Solid Edge part; units mm, degrees
sketch "Sketch1" plane through (0, 0, 0) normal (0, 0, 1) x (1, 0, 0)
  line L0 (0, 0) -> (0, 38.1)
  line L1 (0, 38.1) -> (57.15, 38.1)
  line L2 (57.15, 38.1) -> (57.15, 0)
  line L3 (57.15, 0) -> (0, 0)
  dimension "D1" = 57.15
extrude "Protrusion1" add sketch "Sketch1" along normal blind 9.525
fillet "Round_1" radius 3.175 4 edges at (0, 0, 4.7625) (0, 38.1, 4.7625) (57.15, 38.1, 4.7625) (57.15, 0, 4.7625)
hole "Hole_1" at (50.8, 12.7, 9.525) direction (0, 0, -1) diameter 4.1656 end up to next countersink diameter 9.1186 countersink angle 82
hole "Hole1" at (6.35, 12.7, 9.525) direction (0, 0, -1) diameter 4.1656 end up to next countersink diameter 9.1186 countersink angle 82
hole "Hole_3" at (47.625, 34.29, 9.525) direction (0, 0, -1) diameter 2.1565 end through all
hole "Hole2" at (9.525, 34.29, 9.525) direction (0, 0, -1) diameter 2.1565 end through all
hole "Hole_10" at (50.8, 6.35, 9.525) direction (0, 0, -1) diameter 3.3071 end up to next
hole "Hole3" at (6.35, 6.35, 9.525) direction (0, 0, -1) diameter 3.3071 end up to next
properties material "Polyethylene, low density"
CAD build for the part. Positions are in the model's coordinates, mm. Round coordinates to 2 decimals unless told otherwise and drop trailing zeros. Write each loop counter-clockwise with the first axis right and the second up, starting at its lowest first coordinate (ties: lowest second). Pieces come first, ordered by that corner, then holes. Notation, with made-up numbers: (-25, 58) - (16, 58) arc R38 ccw to (16, 96) - close; hole circle Ø4 at (15, 55.5). An arc over 180 degrees is marked (long way). Return JSON: item names as keys, results as strings. Group by question number.
Item 1: Band-saw the part on D-D on y = 6.35. List the corners of the cut face in (x, z) (3 decimals), plus the area to 3 significant figures.
Item 2: Mould opens along X. For faces 1 (the face through (57.15, 19, 5)), 2 (the face through (0, 19, 5)), 3 (the face through (4.736, 6.708, 4.829)), 4 (the face through (6.44, 14.78, 3.38)) say: +X half, -X half, draft (parallel to the pull), parting line (faces both ways), or undercut.
Item 3: Band-saw the part on A-A on y = 34.29. List the corners of the cut face in (x, z) (3 decimals).
Item 4: Probe probe 1 along X at (y, z) = (34.29, 7.5); probe 2 along X at (y, z) = (6.35, 5.5); probe 3 along Y at (x, z) = (7, 9). List the from-to ranges inside material, lowest first.
Item 5: Band-saw the part on C-C on z = 2. State how many separate pieces and enclosed holes the cut face has, plus the area to 3 significant figures.
Item 6: Flat gauge pins, fed straight in: pin 1 Ø1.3 at (x, y) = (9.525, 34.29) entering from +Z; pin 2 Ø5.5 at (x, y) = (6.35, 12.7) entering from +Z. Where does each tip first touch, or does it go through?
Item 7: Band-saw the part on B-B on x = 6.35. List the corners of the cut face in (y, z) (3 decimals).
Resolved:
{
 "1": {"outline": "(0, 0) - (4.696, 0) - (4.696, 9.525) - (0, 9.525) - close; (8.004, 0) - (49.146, 0) - (49.146, 9.525) - (8.004, 9.525) - close; (52.454, 0) - (57.15, 0) - (57.15, 9.525) - (52.454, 9.525) - close", "area": "481 mm²"},
 "2": {"face 1": "+X half", "face 2": "-X half", "face 3": "undercut", "face 4": "undercut"},
 "3": {"outline": "(0, 0) - (8.447, 0) - (8.447, 9.525) - (0, 9.525) - close; (10.603, 0) - (46.547, 0) - (46.547, 9.525) - (10.603, 9.525) - close; (48.703, 0) - (57.15, 0) - (57.15, 9.525) - (48.703, 9.525) - close"},
 "4": {"probe 1": "x = 0 to 8.45, 10.6 to 46.55, 48.7 to 57.15", "probe 2": "x = 0 to 4.7, 8 to 49.15, 52.45 to 57.15", "probe 3": "y = 0 to 4.83, 7.87 to 8.65, 16.75 to 38.1"},
 "5": {"separate pieces": "1", "enclosed holes": "6", "area": "2,120 mm²"},
 "6": {"pin 1": "passes through", "pin 2": "stops at z = 7.44"},
 "7": {"outline": "(0, 0) - (4.696, 0) - (4.696, 9.525) - (0, 9.525) - close; (8.004, 0) - (10.617, 0) - (10.617, 6.676) - (8.141, 9.525) - (8.004, 9.525) - close; (14.783, 0) - (38.1, 0) - (38.1, 9.525) - (17.259, 9.525) - (14.783, 6.676) - close"}
}
